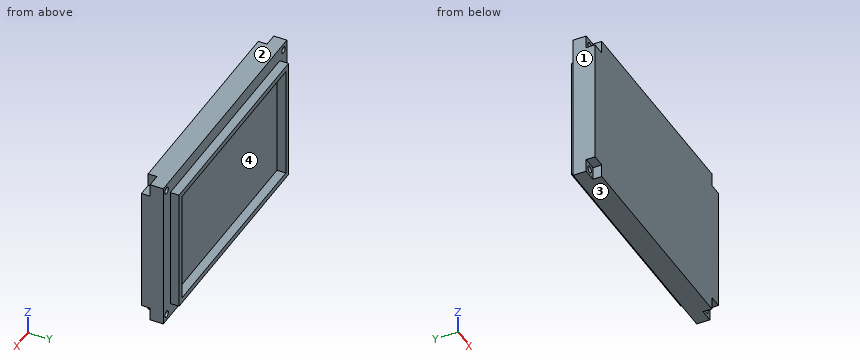
```python
from build123d import *

# Parameters (mm, degrees)
SKETCH1_W               = 139.7
SKETCH1_H               = 88.9
BOSS_EXTRUDE1_DEPTH     = 12.7
SKETCH4_R               = 1.905
CUT_EXTRUDE1_DEPTH      = 84.762252835
MIRROR2_COPY_1_SKETCH_R = 1.905
MIRROR2_COPY_1_DEPTH    = 84.762252835
SKETCH5_W               = 123.825
SKETCH5_H               = 73.025
SKETCH5_W_2             = 117.475
SKETCH5_H_2             = 66.675
BOSS_EXTRUDE2_DEPTH     = 5.08
SKETCH6_W               = 7.62
SKETCH6_H               = 7.62
CUT_EXTRUDE2_DEPTH      = 5.08
MIRROR4_COPY_1_SKETCH_W = 7.62
MIRROR4_COPY_1_SKETCH_H = 7.62
MIRROR4_COPY_1_DEPTH    = 5.08


with BuildPart() as part:
    # Sketch1 → Boss-Extrude1 (new body)
    with BuildSketch(Plane(origin=(0, 0, 0), x_dir=(1, 0, 0), z_dir=(0, 1, 0))):
        Rectangle(SKETCH1_W, SKETCH1_H)
    extrude(amount=BOSS_EXTRUDE1_DEPTH)

    # Sketch4 → Cut-Extrude1 (cut, through all)
    with BuildSketch(Plane(origin=(0, 12.7, 0), x_dir=(1, 0, 0), z_dir=(0, 1, 0))):
        with Locations(Location((-66.04, 40.64, 0), (0, 0, 270))):
            Circle(SKETCH4_R)
    cut_extrude1 = extrude(amount=-CUT_EXTRUDE1_DEPTH, mode=Mode.SUBTRACT)

    # Mirror1: Cut-Extrude1 across plane
    add(cut_extrude1.mirror(Plane(origin=(0, 0, 0), x_dir=(0, 0, 1), z_dir=(1, 0, 0))), mode=Mode.SUBTRACT)

    # Mirror2: Cut-Extrude1 across plane
    add(cut_extrude1.mirror(Plane.XY), mode=Mode.SUBTRACT)

    # Mirror2 copy 1 sketch → Mirror2 copy 1 (cut, through all)
    with BuildSketch(Plane(origin=(0, 12.7, 0), x_dir=(-1, 0, 0), z_dir=(0, 1, 0))):
        with Locations(Location((-66.04, 40.64, 0), (0, 0, 270))):
            Circle(MIRROR2_COPY_1_SKETCH_R)
    extrude(amount=-MIRROR2_COPY_1_DEPTH, mode=Mode.SUBTRACT)

    # Sketch5 → Boss-Extrude2 (add)
    with BuildSketch(Plane(origin=(0, 12.7, 0), x_dir=(1, 0, 0), z_dir=(0, 1, 0))):
        Rectangle(SKETCH5_W, SKETCH5_H)
        Rectangle(SKETCH5_W_2, SKETCH5_H_2, mode=Mode.SUBTRACT)
    extrude(amount=BOSS_EXTRUDE2_DEPTH)

    # Sketch6 → Cut-Extrude2 (cut)
    with BuildSketch(Plane.XZ):
        with Locations((-66.04, 40.64)):
            Rectangle(SKETCH6_W, SKETCH6_H)
    cut_extrude2 = extrude(amount=-CUT_EXTRUDE2_DEPTH, mode=Mode.SUBTRACT)

    # Mirror3: Cut-Extrude2 across plane
    add(cut_extrude2.mirror(Plane(origin=(0, 0, 0), x_dir=(0, 0, 1), z_dir=(1, 0, 0))), mode=Mode.SUBTRACT)

    # Mirror4: Cut-Extrude2 across plane
    add(cut_extrude2.mirror(Plane.XY), mode=Mode.SUBTRACT)

    # Mirror4 copy 1 sketch → Mirror4 copy 1 (cut)
    with BuildSketch(Plane(origin=(0, 0, 0), x_dir=(-1, 0, 0), z_dir=(0, -1, 0))):
        with Locations((-66.04, 40.64)):
            Rectangle(MIRROR4_COPY_1_SKETCH_W, MIRROR4_COPY_1_SKETCH_H)
    extrude(amount=-MIRROR4_COPY_1_DEPTH, mode=Mode.SUBTRACT)


solid = part.part
```
Could you check a few things on this model? Use its own coordinates, in mm. Face numbers are marked on the shaded views. Coordinates: 2 decimals unless noted, no trailing zeros. Loops run counter-clockwise (first coordinate to the right, second up) from the corner with the lowest first, then second, coordinate; pieces in that order, holes last.
1) Will these pins go through, and if not, where does the flat tip stop? pin 1 Ø5.5 at (y, z) = (16, 6) entering from +X; pin 2 Ø1.5 at (x, y) = (65, 2) entering from +Z; pin 3 Ø4 at (x, z) = (-65, 41.5) entering from -Y.
Reported:
pin 1: stops at x = 61.91
pin 2: stops at z = 36.83
pin 3: stops at y = 5.08
2) Please list where these lines run through material, in increasing order: line 1 along X through (y, z) = (7, -40.64) (3 decimals); line 2 along Z through (x, y) = (66.04, 11) (3 decimals).
Reported:
line 1: x = -69.85 to -67.945, -64.135 to 64.135, 67.945 to 69.85
line 2: z = -44.45 to -42.545, -38.735 to 38.735, 42.545 to 44.45
3) Imagine slicing it at B-B (x = 66.04). List the corners of the cut face in (y, z) for me (3 decimals), and give its area (3 significant figures).
Reported:
outline: (0, -36.83) - (5.08, -36.83) - (5.08, -38.735) - (12.7, -38.735) - (12.7, 38.735) - (5.08, 38.735) - (5.08, 36.83) - (0, 36.83) - close; (5.08, -44.45) - (12.7, -44.45) - (12.7, -42.545) - (5.08, -42.545) - close; (5.08, 42.545) - (12.7, 42.545) - (12.7, 44.45) - (5.08, 44.45) - close
area: 994 mm2
4) Thinking about a two-plate mould opening in Z: for the marked faces 1, 2, 3 and 4, which applies, released by +Z, released by -Z, zero draft, split by the parting line, or undercut?
Reported:
face 1: zero draft
face 2: released by +Z
face 3: released by -Z
face 4: undercut
5) Imagine slicing it at A-A (z = -40.64). List the corners of the cut face in (x, y) for me (3 decimals).
Reported:
outline: (-69.85, 5.08) - (-67.945, 5.08) - (-67.945, 12.7) - (-69.85, 12.7) - close; (-64.135, 5.08) - (-62.23, 5.08) - (-62.23, 0) - (62.23, 0) - (62.23, 5.08) - (64.135, 5.08) - (64.135, 12.7) - (-64.135, 12.7) - close; (67.945, 5.08) - (69.85, 5.08) - (69.85, 12.7) - (67.945, 12.7) - close
6) Imagine slicing it at C-C (y = 14.25). List the corners of the cut face in (x, z) for me.
Reported:
outline: (-61.91, -36.51) - (61.91, -36.51) - (61.91, 36.51) - (-61.91, 36.51) - close; hole (-58.74, -33.34) - (58.74, -33.34) - (58.74, 33.34) - (-58.74, 33.34) - close
7) Imagine slicing it at D-D (z = -17). List the corners of the cut face in (x, y) for me.
Reported:
outline: (-69.85, 0) - (69.85, 0) - (69.85, 12.7) - (61.91, 12.7) - (61.91, 17.78) - (58.74, 17.78) - (58.74, 12.7) - (-58.74, 12.7) - (-58.74, 17.78) - (-61.91, 17.78) - (-61.91, 12.7) - (-69.85, 12.7) - close
